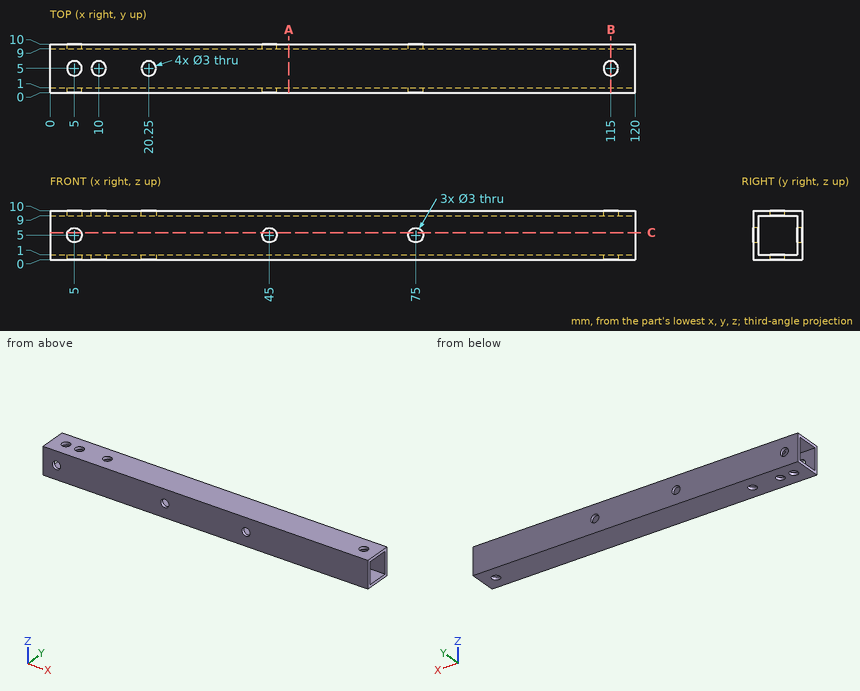
The figure shows three views and two pictorial views of one solid part (mm, origin at its lowest corner). Answer the questions. Round coordinates to 2 decimals unless told otherwise and drop trailing zeros. Order: outer loops, then holes, each group sorted by start corner. A loop starts at its lowest first (then second) coordinate and runs counter-clockwise, first axis right, second up. Notation, with made-up numbers: (53, -7) - (86, -7) arc R10 ccw to (86, 11) - close; hole circle Ø6 at (-7.5, -35). An arc over 180 degrees is marked (long way). Write item = value, one per line. Start each with the question number.
1) Section C-C, the plane z = 5.5 is taken. Count the separate pieces of the cut face and the enclosed holes in it, plus the area to 3 significant figures.
2) Section B-B, the plane x = 115 is taken. Write down the section's boundary in (y, z), plus the area to 3 significant figures.
3) Straight lines are drawn through the part: L1, parallel to X at y = 0.65, z = 5; L2, parallel to Z at x = 77.5, y = 8.25. For each, find the intervals that lie inside material, in ascending order.
4) Section A-A, the plane x = 49 is taken. Write down the section's boundary in (y, z), plus the area to 3 significant figures.
Results list:
q1.separate_pieces = 8
q1.enclosed_holes = 0
q1.area = 223 mm^2
q2.outline = (0, 0) - (3.5, 0) - (3.5, 1) - (1, 1) - (1, 9) - (3.5, 9) - (3.5, 10) - (0, 10) - close; (6.5, 0) - (10, 0) - (10, 10) - (6.5, 10) - (6.5, 9) - (9, 9) - (9, 1) - (6.5, 1) - close
q2.area = 30.0 mm^2
q3.L1 = 0 to 3.5, 6.5 to 43.5, 46.5 to 73.5, 76.5 to 120
q3.L2 = 0 to 1, 9 to 10
q4.outline = (0, 0) - (10, 0) - (10, 10) - (0, 10) - close; hole (1, 1) - (9, 1) - (9, 9) - (1, 9) - close
q4.area = 36.0 mm^2
